Source: CAD feature listing. Evaluate the final solid. Frame: model axes, mm. Round coordinates to 2 decimals unless told otherwise and drop trailing zeros. Order: outer loops, then holes, each group sorted by start corner. A loop starts at its lowest first (then second) coordinate and runs counter-clockwise, first axis right, second up. Notation, with made-up numbers: (82.5, 46.5) -> (129.5, 46.5) arc R25 ccw to (129.5, 60.5) -> close; hole circle Ø9 at (3, 58). An arc over 180 degrees is marked (long way). One line per item, written item: value. Start each with the question number.
1) Section B-B (x = 47). Return the cut outline in (y, z).
2) Ray query, L1, parallel to X at y = -24, z = 4.1; L2, parallel to X at y = -24, z = 1.4; L3, parallel to X at y = 77, z = 4.55. Return the intervals inside material, ascending.
3) Pin query (flat end, axial travel): P1, Ø1, axis at x = -45, z = 4, coming from the -Y side; P2, Ø3, axis at y = -71, z = 4, coming from the -X side; P3, Ø1, axis at x = -64, z = 3.5, coming from the -Y side. Return the tip coordinate at first contact, or that it passes through.
4) Section A-A (z = 2). Return the cut outline in (x, y).
5) Section C-C (y = -71.5). Return the cut outline in (x, z).
```python
from build123d import *

# Parameters (mm, degrees)
PAD_DEPTH    = 5
POCKET_DEPTH = 3
SKETCH004_R  = 0.8
HOLE_DEPTH   = 25


with BuildPart() as part:
    # Sketch → Pad (new body)
    with BuildSketch(Plane.XY):
        Polygon((86.60254, -50), (86.60254, 50), (0, 100), (-86.60254, 50), (-86.60254, -50), (0, -100), align=None)
    extrude(amount=PAD_DEPTH)

    # Sketch003 (on Face7 of Pad) → Pocket (cut)
    with BuildSketch(Plane(origin=(0, 0, 0), x_dir=(1, 0, 0), z_dir=(0, 0, -1))):
        with BuildLine():
            ThreePointArc((82.208138, 20.772506), (85.73254, 24), (82.208138, 27.227494))
            Line((67.51225, 25.932512), (82.208138, 27.227494))
            ThreePointArc((67.51225, 25.932512), (65.74254, 24), (67.51225, 22.067488))
            Line((67.51225, 22.067488), (82.208138, 20.772506))
        make_face()
    extrude(amount=-POCKET_DEPTH, mode=Mode.SUBTRACT)

    # Sketch004 (on Face13 of Pocket) → Hole (cut)
    with BuildSketch(Plane(origin=(0, 0, 3), x_dir=(1, 0, 0), z_dir=(0, 0, -1))):
        with Locations((67.21254, 24)):
            Circle(SKETCH004_R)
        with Locations((70.78254, 24)):
            Circle(SKETCH004_R)
        with Locations((74.35254, 24)):
            Circle(SKETCH004_R)
    extrude(amount=-HOLE_DEPTH, mode=Mode.SUBTRACT)


solid = part.part
```
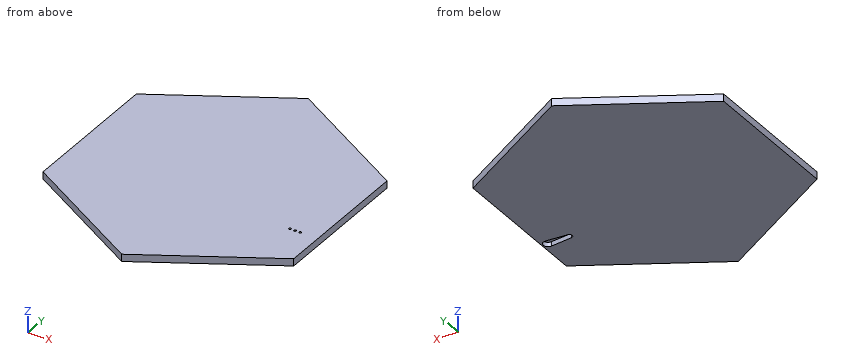
Findings:
1. outline: (-72.86, 0) -> (72.86, 0) -> (72.86, 5) -> (-72.86, 5) -> close
2. L1: -86.6 to 66.41, 68.01 to 69.98, 71.58 to 73.55, 75.15 to 86.6
2. L2: -86.6 to 65.74, 85.73 to 86.6
2. L3: -39.84 to 39.84
3. P1: y = -74.31
3. P2: x = -52.83
3. P3: y = -63.34
4. outline: (-86.6, -50) -> (0, -100) -> (86.6, -50) -> (86.6, 50) -> (0, 100) -> (-86.6, 50) -> close; hole (67.51, -25.93) -> (82.21, -27.23) arc R3.24 ccw (long way) to (82.21, -20.77) -> (67.51, -22.07) arc R1.94 ccw to start
5. outline: (-49.36, 0) -> (49.36, 0) -> (49.36, 5) -> (-49.36, 5) -> close
